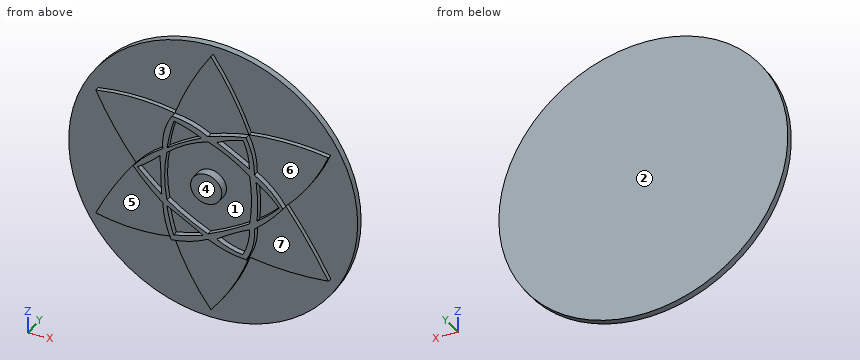
from build123d import *

# Parameters (mm, degrees)
F2_R     = 3.597318
F3_DEPTH = 4.572
F1_R     = 33.297868
F4_DEPTH = 1.524
F6_DEPTH = 2.286
F7_DEPTH = 1.016


with BuildPart() as f3:
    # F2 (on face) → F3 (new body)
    with BuildSketch(Plane.XZ):
        Circle(F2_R)
    extrude(amount=F3_DEPTH)

    # F1 (on Front) → F4 (join)
    with BuildSketch(Plane.XZ):
        Circle(F1_R)
    extrude(amount=F4_DEPTH)

    # F5 (on face) → F6 (join)
    with BuildSketch(Plane.XZ.offset(1.524)):
        with BuildLine():
            ThreePointArc((10.713429, 6.318242), (10.248964, 10.715615), (8.788303, 14.889233))
            ThreePointArc((8.788303, 14.889233), (4.333719, 13.860328), (0, 12.40402))
            ThreePointArc((0, 12.40402), (-3.998899, 14.133336), (-8.289627, 14.889233))
            ThreePointArc((-8.289627, 14.889233), (-10.051786, 10.753928), (-10.412228, 6.273299))
            ThreePointArc((-10.412228, 6.273299), (-14.092567, 3.413894), (-17.265329, 0))
            ThreePointArc((-17.265329, 0), (-14.001547, -3.668596), (-10.406789, -7.01353))
            ThreePointArc((-10.406789, -7.01353), (-9.830191, -11.331497), (-8.465515, -15.468521))
            ThreePointArc((-8.465515, -15.468521), (-4.093198, -14.52777), (0, -12.725577))
            ThreePointArc((0, -12.725577), (4.302612, -14.348925), (8.847156, -15.052379))
            ThreePointArc((8.847156, -15.052379), (10.398679, -11.127024), (10.702084, -6.917085))
            ThreePointArc((10.702084, -6.917085), (14.203553, -3.658977), (17.283723, 0))
            ThreePointArc((17.283723, 0), (14.361308, 3.536323), (10.713429, 6.318242))
        make_face()
        with BuildLine():
            ThreePointArc((-10.74901, -4.952658), (-13.534815, -2.529093), (-16.22518, 0))
            ThreePointArc((-16.22518, 0), (-13.56313, 2.052862), (-11.09127, 4.331163))
            ThreePointArc((-11.09127, 4.331163), (-10.819822, -0.307049), (-10.74901, -4.952658))
        make_face(mode=Mode.SUBTRACT)
        with BuildLine():
            ThreePointArc((-1.113919, -12.127829), (-4.506024, -13.201244), (-7.931484, -14.162923))
            ThreePointArc((-7.931484, -14.162923), (-8.823734, -10.821527), (-9.457804, -7.421674))
            ThreePointArc((-9.457804, -7.421674), (-5.253039, -9.716557), (-1.113919, -12.127829))
        make_face(mode=Mode.SUBTRACT)
        with BuildLine():
            ThreePointArc((9.610696, -5.973405), (4.908164, -8.877536), (0, -11.418739))
            ThreePointArc((0, -11.418739), (-4.882883, -8.963516), (-9.457804, -5.973405))
            ThreePointArc((-9.457804, -5.973405), (-9.979883, -0.165049), (-9.457804, 5.643307))
            ThreePointArc((-9.457804, 5.643307), (-5.012545, 8.890946), (0, 11.167321))
            ThreePointArc((0, 11.167321), (5.044159, 8.820798), (9.610696, 5.643307))
            ThreePointArc((9.610696, 5.643307), (10.039267, -0.165049), (9.610696, -5.973405))
        make_face(mode=Mode.SUBTRACT)
        with BuildLine():
            ThreePointArc((9.632519, -7.387693), (9.220737, -10.79398), (8.049564, -14.018993))
            ThreePointArc((8.049564, -14.018993), (4.925761, -13.364903), (2.01722, -12.050994))
            ThreePointArc((2.01722, -12.050994), (5.719103, -9.546625), (9.632519, -7.387693))
        make_face(mode=Mode.SUBTRACT)
        with BuildLine():
            ThreePointArc((11.104458, 4.606938), (13.937738, 2.51162), (16.409498, 0))
            ThreePointArc((16.409498, 0), (13.995151, -2.521496), (11.318372, -4.762447))
            ThreePointArc((11.318372, -4.762447), (11.437982, -0.072581), (11.104458, 4.606938))
        make_face(mode=Mode.SUBTRACT)
        with BuildLine():
            ThreePointArc((-9.457804, 6.745422), (-8.765935, 10.318411), (-7.858452, 13.842813))
            ThreePointArc((-7.858452, 13.842813), (-4.608306, 12.909868), (-1.483598, 11.617566))
            ThreePointArc((-1.483598, 11.617566), (-5.574191, 9.350874), (-9.457804, 6.745422))
        make_face(mode=Mode.SUBTRACT)
        with BuildLine():
            ThreePointArc((8.106259, 13.965921), (9.19576, 10.788913), (9.540202, 7.447992))
            ThreePointArc((9.540202, 7.447992), (5.829565, 9.586664), (2.058865, 11.617566))
            ThreePointArc((2.058865, 11.617566), (4.983842, 13.045962), (8.106259, 13.965921))
        make_face(mode=Mode.SUBTRACT)
    extrude(amount=F6_DEPTH)

    # F5 (on face) → F7 (join)
    with BuildSketch(Plane.XZ.offset(1.524)):
        with BuildLine():
            ThreePointArc((-10.412228, 6.273299), (-10.051786, 10.753928), (-8.289627, 14.889233))
            ThreePointArc((-8.289627, 14.889233), (-17.405207, 15.756847), (-26.520787, 14.889233))
            ThreePointArc((-26.520787, 14.889233), (-22.28618, 7.200243), (-17.265329, 0))
            ThreePointArc((-17.265329, 0), (-14.092567, 3.413894), (-10.412228, 6.273299))
        make_face()
        with BuildLine():
            ThreePointArc((0, 12.40402), (4.333719, 13.860328), (8.788303, 14.889233))
            ThreePointArc((8.788303, 14.889233), (4.902081, 23.371612), (0, 31.31032))
            ThreePointArc((0, 31.31032), (-4.677616, 23.368743), (-8.289627, 14.889233))
            ThreePointArc((-8.289627, 14.889233), (-3.998899, 14.133336), (0, 12.40402))
        make_face()
        with BuildLine():
            ThreePointArc((27.086085, 14.889233), (17.937194, 15.570442), (8.788303, 14.889233))
            ThreePointArc((8.788303, 14.889233), (10.248964, 10.715615), (10.713429, 6.318242))
            ThreePointArc((10.713429, 6.318242), (14.361308, 3.536323), (17.283723, 0))
            ThreePointArc((17.283723, 0), (22.902766, 6.97201), (27.086085, 14.889233))
        make_face()
        with BuildLine():
            ThreePointArc((27.086085, -15.368001), (22.47422, -7.499462), (17.283723, 0))
            ThreePointArc((17.283723, 0), (14.203553, -3.658977), (10.702084, -6.917085))
            ThreePointArc((10.702084, -6.917085), (10.398679, -11.127024), (8.847156, -15.052379))
            ThreePointArc((8.847156, -15.052379), (17.955268, -15.866193), (27.086085, -15.368001))
        make_face()
        with BuildLine():
            ThreePointArc((0, -30.730024), (5.16221, -23.308024), (8.847156, -15.052379))
            ThreePointArc((8.847156, -15.052379), (4.302612, -14.348925), (0, -12.725577))
            ThreePointArc((0, -12.725577), (-4.093198, -14.52777), (-8.465515, -15.468521))
            ThreePointArc((-8.465515, -15.468521), (-4.799827, -23.413825), (0, -30.730024))
        make_face()
        with BuildLine():
            ThreePointArc((-10.406789, -7.01353), (-14.001547, -3.668596), (-17.265329, 0))
            ThreePointArc((-17.265329, 0), (-22.318324, -7.35541), (-26.520787, -15.227773))
            ThreePointArc((-26.520787, -15.227773), (-17.506335, -16.336903), (-8.465515, -15.468521))
            ThreePointArc((-8.465515, -15.468521), (-9.830191, -11.331497), (-10.406789, -7.01353))
        make_face()
        with BuildLine():
            ThreePointArc((-9.457804, -7.421674), (-8.823734, -10.821527), (-7.931484, -14.162923))
            ThreePointArc((-7.931484, -14.162923), (-4.506024, -13.201244), (-1.113919, -12.127829))
            ThreePointArc((-1.113919, -12.127829), (-5.253039, -9.716557), (-9.457804, -7.421674))
        make_face()
        with BuildLine():
            ThreePointArc((2.01722, -12.050994), (4.925761, -13.364903), (8.049564, -14.018993))
            ThreePointArc((8.049564, -14.018993), (9.220737, -10.79398), (9.632519, -7.387693))
            ThreePointArc((9.632519, -7.387693), (5.719103, -9.546625), (2.01722, -12.050994))
        make_face()
        with BuildLine():
            ThreePointArc((-9.457804, -5.973405), (-4.882883, -8.963516), (0, -11.418739))
            ThreePointArc((0, -11.418739), (4.908164, -8.877536), (9.610696, -5.973405))
            ThreePointArc((9.610696, -5.973405), (10.039267, -0.165049), (9.610696, 5.643307))
            ThreePointArc((9.610696, 5.643307), (5.044159, 8.820798), (0, 11.167321))
            ThreePointArc((0, 11.167321), (-5.012545, 8.890946), (-9.457804, 5.643307))
            ThreePointArc((-9.457804, 5.643307), (-9.979883, -0.165049), (-9.457804, -5.973405))
        make_face()
        with BuildLine():
            ThreePointArc((11.318372, -4.762447), (13.995151, -2.521496), (16.409498, 0))
            ThreePointArc((16.409498, 0), (13.937738, 2.51162), (11.104458, 4.606938))
            ThreePointArc((11.104458, 4.606938), (11.437982, -0.072581), (11.318372, -4.762447))
        make_face()
        with BuildLine():
            ThreePointArc((-1.483598, 11.617566), (-4.608306, 12.909868), (-7.858452, 13.842813))
            ThreePointArc((-7.858452, 13.842813), (-8.765935, 10.318411), (-9.457804, 6.745422))
            ThreePointArc((-9.457804, 6.745422), (-5.574191, 9.350874), (-1.483598, 11.617566))
        make_face()
        with BuildLine():
            ThreePointArc((2.058865, 11.617566), (5.829565, 9.586664), (9.540202, 7.447992))
            ThreePointArc((9.540202, 7.447992), (9.19576, 10.788913), (8.106259, 13.965921))
            ThreePointArc((8.106259, 13.965921), (4.983842, 13.045962), (2.058865, 11.617566))
        make_face()
        with BuildLine():
            ThreePointArc((-11.09127, 4.331163), (-13.56313, 2.052862), (-16.22518, 0))
            ThreePointArc((-16.22518, 0), (-13.534815, -2.529093), (-10.74901, -4.952658))
            ThreePointArc((-10.74901, -4.952658), (-10.819822, -0.307049), (-11.09127, 4.331163))
        make_face()
    extrude(amount=F7_DEPTH)


solid = f3.part
Check sheet for the modelled part. Datum: model origin and axes. Units: mm. Face numbers are marked on the shaded views. A direction names the side the tool comes from. Give positions to 0.01 mm unless a question says otherwise; leave off trailing zeros. Write each loop counter-clockwise with the first axis right and the second up, starting at its lowest first coordinate (ties: lowest second). Pieces come first, ordered by that corner, then holes. Notation, with made-up numbers: (-24, 30) -> (-6, 30) arc R19 cw to (-6, 63) -> close; hole circle Ø2 at (54.5, 24.25). An arc over 180 degrees is marked (long way). Use one line per item in the form item = value. Start each with the question number.
1. Section check A-A (x = -24.5). Record the cut outline in (y, z).
2. Go/stop test with flat-tipped pins: P1, Ø2, axis at x = -3.5, z = 10, coming from the -Y side; P2, Ø12.5, axis at x = -21, z = 6, coming from the -Y side; P3, Ø5, axis at x = 24.5, z = 4.5, coming from the -Y side. Record where each tip stops, or that it passes through.
3. Section check B-B (y = -0.7). Record the cut outline in (x, z), and give its area (3 significant figures).
4. Section check D-D (x = 1). Record the cut outline in (y, z).
5. Access from +Z, -Z, +X, -X, +Y, -Y to the whole of each face (thin tool, end or side, straight path). Record for the marked faces 4, 5, 6 and 7.
6. Section check C-C (z = -20). Record the cut outline in (x, y), and give its area (3 significant figures).
7. Thickness scan on line 1 along X through (y, z) = (-3.75, 9); line 2 along Y through (x, z) = (-2.5, 28); line 3 along X through (y, z) = (-2.6, -6). Record the ranges inside material, lowest first. Write a range as from..to.
8. Mould release check, pull along Z, two halves, no side actions. Record for the marked faces 1, 2 and 3: pulls with the +Z half, pulls with the -Z half, needs draft (parallel to the pull), parting line crosses it, or undercut.
Conclusion:
q1.outline = (-2.54, -15.65) -> (-1.52, -15.65) -> (-1.52, -22.55) -> (0, -22.55) -> (0, 22.55) -> (-1.52, 22.55) -> (-1.52, 15.23) -> (-2.54, 15.23) -> (-2.54, 10.98) -> (-1.52, 10.98) -> (-1.52, -11.18) -> (-2.54, -11.18) -> close
q2.P1 = -3.81
q2.P2 = -2.54
q2.P3 = -1.52
q3.outline = circle Ø66.6 at (0, 0)
q3.area = 3,480 mm²
q4.outline = (-4.57, -3.46) -> (-2.54, -3.46) -> (-2.54, -10.94) -> (-3.81, -10.94) -> (-3.81, -13.2) -> (-2.54, -13.2) -> (-2.54, -29.51) -> (-1.52, -29.51) -> (-1.52, -33.28) -> (0, -33.28) -> (0, 33.28) -> (-1.52, 33.28) -> (-1.52, 29.86) -> (-2.54, 29.86) -> (-2.54, 12.78) -> (-3.81, 12.78) -> (-3.81, 10.78) -> (-2.54, 10.78) -> (-2.54, 3.46) -> (-4.57, 3.46) -> close
q5.face_4 = +Z, -Z, +X, -X, -Y
q5.face_5 = -Z, -X, -Y
q5.face_6 = +Z, +X, -Y
q5.face_7 = -Z, +X, -Y
q6.outline = (-26.62, -1.52) -> (-6.55, -1.52) -> (-6.55, -2.54) -> (6.86, -2.54) -> (6.86, -1.52) -> (26.62, -1.52) -> (26.62, 0) -> (-26.62, 0) -> close
q6.area = 94.8 mm²
q7.line_1 = -10.37..-9.05, -6.14..-4.82, 4.73..6.87, 9.48..10.55
q7.line_2 = -1.52..0
q7.line_3 = -11.57..-9.42, 9.57..11.78
q8.face_1 = undercut
q8.face_2 = needs draft
q8.face_3 = undercut
